Can you work these out from the model? Positions are in its coordinate system, mm. Give positions to 0.01 mm unless a question says otherwise; leave off trailing zeros. Answer as CSV lines item,"result". Start each with the question number.
1. If we section it at A-A on z = 387: Count the separate pieces of the cut face and the enclosed holes in it, plus the area to 3 significant figures.
2. I'm going to push flat-ended pins straight in: P1, Ø4, axis at x = 3.5, z = 79, coming from the +Y side; P2, Ø0.5, axis at y = -13.5, z = 429, coming from the -X side; P3, Ø0.5, axis at x = -4.5, z = 148, coming from the -Y side; P4, Ø1.1, axis at y = 4.5, z = 183, coming from the -X side. Where does each tip first touch, or does it pass through?
3. I need wall thicknesses on line 1 (Y direction, x = 12, z = 172); line 2 (Z direction, x = 0, y = -4.2). Which ranges of each line are inside material? Lowest first, please. Write a range as [from, to].
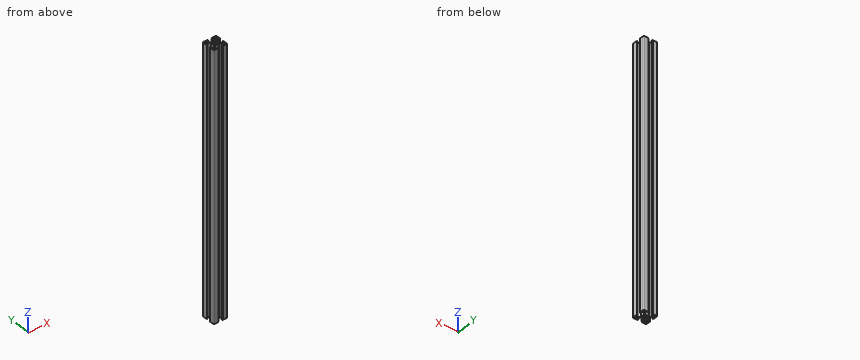
```python
from build123d import *

# Parameters (mm, degrees)
SKETCH_1_W                       = 4
SKETCH_1_H                       = 4
EXTRUDE_1_DEPTH                  = 580
FILLET_1_R                       = 1
FILLET_2_R                       = 2
FILLET_3_R                       = 0.5
PATTERN_CIRCULAR_1_COUNT         = 4
FILLET_1_OF_PATTERN_CIRCULAR_1_R = 1
FILLET_2_OF_PATTERN_CIRCULAR_1_R = 2
FILLET_3_OF_PATTERN_CIRCULAR_1_R = 0.5
SKETCH_2_R                       = 3.4
CUT_EXTRUDE_1_DEPTH              = 581
SKETCH_3_R                       = 2.6
CUT_EXTRUDE_2_DEPTH              = 10


with BuildPart() as part:
    # 草图1 → 凸台-拉伸1 (new body)
    with BuildSketch(Plane.XY):
        Polygon((5.7, 0), (5.7, 4.427207794), (9.672792206, 8.4), (13.2, 8.4), (13.2, 4.1), (14.1, 4.1), (14.1, 5.1), (15, 5.1), (15, 15), (5.1, 15), (5.1, 14.1), (4.1, 14.1), (4.1, 13.2), (8.4, 13.2), (8.4, 9.672792206), (4.427207794, 5.7), (0, 5.7), (0, 0), align=None)
        with Locations((11.7, 11.7)):
            Rectangle(SKETCH_1_W, SKETCH_1_H, mode=Mode.SUBTRACT)
    extrude_1 = extrude(amount=EXTRUDE_1_DEPTH)

    # 圆角1
    fillet_1_edges = [part.edges().sort_by_distance(p)[0] for p in [
        (13.7, 9.7, 290),
        (13.7, 13.7, 290),
        (9.7, 13.7, 290),
        (9.7, 9.7, 290),
    ]]
    fillet(fillet_1_edges, radius=FILLET_1_R)

    # 圆角2
    fillet_2_edges = [part.edges().sort_by_distance(p)[0] for p in [
        (15, 15, 290),
    ]]
    fillet(fillet_2_edges, radius=FILLET_2_R)

    # 圆角3
    fillet_3_edges = [part.edges().sort_by_distance(p)[0] for p in [
        (4.427207794, 5.7, 290),
        (8.4, 9.672792206, 290),
        (8.4, 13.2, 290),
        (13.2, 8.4, 290),
        (9.672792206, 8.4, 290),
        (5.7, 4.427207794, 290),
    ]]
    fillet(fillet_3_edges, radius=FILLET_3_R)

    # 阵列(圆周)1: 凸台-拉伸1 ×4 about axis
    pattern_circular_1_axis = Axis((0, 0, 0), (0, 0, 1))
    for i in range(1, PATTERN_CIRCULAR_1_COUNT):
        add(extrude_1.rotate(pattern_circular_1_axis, i * 360 / PATTERN_CIRCULAR_1_COUNT))

    # 圆角1 of 阵列(圆周)1
    fillet_1_of_pattern_circular_1_edges = [part.edges().sort_by_distance(p)[0] for p in [
        (-9.7, 13.7, 290),
        (-13.7, 13.7, 290),
        (-13.7, 9.7, 290),
        (-9.7, 9.7, 290),
        (-13.7, -9.7, 290),
        (-13.7, -13.7, 290),
        (-9.7, -13.7, 290),
        (-9.7, -9.7, 290),
        (9.7, -13.7, 290),
        (13.7, -13.7, 290),
        (13.7, -9.7, 290),
        (9.7, -9.7, 290),
    ]]
    fillet(fillet_1_of_pattern_circular_1_edges, radius=FILLET_1_OF_PATTERN_CIRCULAR_1_R)

    # 圆角2 of 阵列(圆周)1
    fillet_2_of_pattern_circular_1_edges = [part.edges().sort_by_distance(p)[0] for p in [
        (-15, 15, 290),
        (-15, -15, 290),
        (15, -15, 290),
    ]]
    fillet(fillet_2_of_pattern_circular_1_edges, radius=FILLET_2_OF_PATTERN_CIRCULAR_1_R)

    # 圆角3 of 阵列(圆周)1
    fillet_3_of_pattern_circular_1_edges = [part.edges().sort_by_distance(p)[0] for p in [
        (-5.7, 4.427207794, 290),
        (-9.672792206, 8.4, 290),
        (-13.2, 8.4, 290),
        (-8.4, 13.2, 290),
        (-8.4, 9.672792206, 290),
        (-4.427207794, 5.7, 290),
        (-4.427207794, -5.7, 290),
        (-8.4, -9.672792206, 290),
        (-8.4, -13.2, 290),
        (-13.2, -8.4, 290),
        (-9.672792206, -8.4, 290),
        (-5.7, -4.427207794, 290),
        (5.7, -4.427207794, 290),
        (9.672792206, -8.4, 290),
        (13.2, -8.4, 290),
        (8.4, -13.2, 290),
        (8.4, -9.672792206, 290),
        (4.427207794, -5.7, 290),
    ]]
    fillet(fillet_3_of_pattern_circular_1_edges, radius=FILLET_3_OF_PATTERN_CIRCULAR_1_R)

    # 草图2 → 切除-拉伸1 (cut, through all)
    with BuildSketch(Plane.XY.offset(580)):
        Circle(SKETCH_2_R)
    extrude(amount=-CUT_EXTRUDE_1_DEPTH, mode=Mode.SUBTRACT)

    # 草图3 → 切除-拉伸2 (cut, symmetric)
    with BuildSketch(Plane(origin=(0, 0, 0), x_dir=(1, 0, 0), z_dir=(0, 1, 0))):
        with Locations((0, -30)):
            Circle(SKETCH_3_R)
        with Locations((0, -90)):
            Circle(SKETCH_3_R)
    extrude(amount=CUT_EXTRUDE_2_DEPTH, both=True, mode=Mode.SUBTRACT)


solid = part.part
```
Computed values:
1,separate pieces,"1"
1,enclosed holes,"5"
1,area,"293 mm2"
2,P1,"stops at y = 15"
2,P2,"stops at x = -14.98"
2,P3,"stops at y = -14.1"
2,P4,"stops at x = -14.1"
3,line 1,"y = [-15, -13.7], [-9.7, -8.4], [8.4, 9.7], [13.7, 15]"
3,line 2,"z = [0, 27.4], [32.6, 87.4], [92.6, 580]"
